```python
from build123d import *

# Parameters (mm, degrees)
SKETCH1_W           = 30
SKETCH1_H           = 42
BOSS_EXTRUDE1_DEPTH = 13.5
SKETCH2_R           = 11
CUT_EXTRUDE1_DEPTH  = 38.349698794
SKETCH3_R           = 1.9
CUT_EXTRUDE2_DEPTH  = 10
SKETCH7_W           = 27
SKETCH7_H           = 42
BOSS_EXTRUDE2_DEPTH = 4.4
SKETCH6_R           = 1.9
CUT_EXTRUDE3_DEPTH  = 10
FILLET1_R           = 10


with BuildPart() as part:
    # Sketch1 → Boss-Extrude1 (new, symmetric)
    with BuildSketch(Plane.XY):
        Rectangle(SKETCH1_W, SKETCH1_H)
    extrude(amount=BOSS_EXTRUDE1_DEPTH, both=True)

    # Sketch2 → Cut-Extrude1 (cut, through all)
    with BuildSketch(Plane.XY.offset(13.5)):
        Circle(SKETCH2_R)
    extrude(amount=-CUT_EXTRUDE1_DEPTH, mode=Mode.SUBTRACT)

    # Sketch3 → Cut-Extrude2 (cut)
    with BuildSketch(Plane.XY.offset(13.5)):
        with Locations((-11.313708499, 11.313708499)):
            Circle(SKETCH3_R)
        with Locations((0, 16)):
            Circle(SKETCH3_R)
        with Locations((11.313708499, 11.313708499)):
            Circle(SKETCH3_R)
        with Locations((11.313708499, -11.313708499)):
            Circle(SKETCH3_R)
        with Locations((0, -16)):
            Circle(SKETCH3_R)
        with Locations((-11.313708499, -11.313708499)):
            Circle(SKETCH3_R)
    extrude(amount=-CUT_EXTRUDE2_DEPTH, mode=Mode.SUBTRACT)

    # Sketch7 → Boss-Extrude2 (add)
    with BuildSketch(Plane(origin=(15, 0, 0), x_dir=(0, 0, -1), z_dir=(1, 0, 0))):
        Rectangle(SKETCH7_W, SKETCH7_H)
    extrude(amount=BOSS_EXTRUDE2_DEPTH)

    # Sketch6 → Cut-Extrude3 (cut)
    with BuildSketch(Plane(origin=(19.4, 0, 0), x_dir=(0, 0, -1), z_dir=(1, 0, 0))):
        with Locations((9.5, 17)):
            Circle(SKETCH6_R)
        with Locations((-9.5, 17)):
            Circle(SKETCH6_R)
        with Locations((9.5, -17)):
            Circle(SKETCH6_R)
        with Locations((-9.5, -17)):
            Circle(SKETCH6_R)
    extrude(amount=-CUT_EXTRUDE3_DEPTH, mode=Mode.SUBTRACT)

    # Fillet1
    fillet1_edges = [part.edges().sort_by_distance(p)[0] for p in [
        (-15, -21, 0),
        (-15, 21, 0),
    ]]
    fillet(fillet1_edges, radius=FILLET1_R)


solid = part.part
```
Verification items for the finished model (mm, model axes). A direction names the side the tool comes from. Coordinates: 2 decimals unless noted, no trailing zeros. Loops run counter-clockwise (first coordinate to the right, second up) from the corner with the lowest first, then second, coordinate; pieces in that order, holes last. Notation, with made-up numbers: (69, -6.5) - (110, -6.5) arc R19 ccw to (110, 9.5) - close; hole circle Ø3 at (58, -23). An arc over 180 degrees is marked (long way). Answer as a JSON object with one key per item and string values.
(1) Mould release check, pull along Y, two halves, no side actions. Record for faces 4 (the cylindrical face through (-0.247, 17.884, 8.57)), 5 (the flat face through (-15, 0, 0)), 6 (the cylindrical face through (-12.15, -17.99, 0.19)): pulls with the +Y half, pulls with the -Y half, needs draft (parallel to the pull), parting line crosses it, or undercut.
Response:
{"face 4": "undercut", "face 5": "needs draft", "face 6": "pulls with the -Y half"}
(2) Cross-section at A-A, the plane y = 0. Record the boundary of the cut face in (x, z).
Response:
{"outline": "(-15, -13.5) - (-11, -13.5) - (-11, 13.5) - (-15, 13.5) - close; (11, -13.5) - (19.4, -13.5) - (19.4, 13.5) - (11, 13.5) - close"}
(3) Cross-section at B-B, the plane z = -9.5. Record the boundary of the cut face in (x, y).
Response:
{"outline": "(-15, -11) arc R10 ccw to (-5, -21) - (19.4, -21) - (19.4, -18.9) - (9.4, -18.9) - (9.4, -15.1) - (19.4, -15.1) - (19.4, 15.1) - (9.4, 15.1) - (9.4, 18.9) - (19.4, 18.9) - (19.4, 21) - (-5, 21) arc R10 ccw to (-15, 11) - close; hole circle Ø22 at (0, 0)"}
(4) Cross-section at D-D, the plane x = 12. Record the boundary of the cut face in (y, z).
Response:
{"outline": "(-21, -13.5) - (21, -13.5) - (21, 13.5) - (13.09, 13.5) - (13.09, 3.5) - (9.54, 3.5) - (9.54, 13.5) - (-9.54, 13.5) - (-9.54, 3.5) - (-13.09, 3.5) - (-13.09, 13.5) - (-21, 13.5) - close; hole circle Ø3.8 at (-17, -9.5); hole circle Ø3.8 at (-17, 9.5); hole circle Ø3.8 at (17, -9.5); hole circle Ø3.8 at (17, 9.5)"}
(5) Cross-section at C-C, the plane x = 0. Record the boundary of the cut face in (y, z), then the cut area to 3 significant figures.
Response:
{"outline": "(-21, -13.5) - (-11, -13.5) - (-11, 13.5) - (-14.1, 13.5) - (-14.1, 3.5) - (-17.9, 3.5) - (-17.9, 13.5) - (-21, 13.5) - close; (11, -13.5) - (21, -13.5) - (21, 13.5) - (17.9, 13.5) - (17.9, 3.5) - (14.1, 3.5) - (14.1, 13.5) - (11, 13.5) - close", "area": "464 mm²"}
(6) Access from +Z, -Z, +X, -X, +Y, -Y to the whole of each face (thin tool, end or side, straight path). Record for faces 1 (the cylindrical face through (-9.559, 10.586, 8.57)), 2 (the cylindrical face through (14.47, -15.398, -10.521)), 3 (the flat face through (6, -10, 13.5)).
Response:
{"face 1": "+Z", "face 2": "+X", "face 3": "+Z, +X, -X, +Y, -Y"}
(7) Scan lines: line 1 along Y through (x, z) = (10, 9.75); line 2 along X through (y, z) = (12, 4); line 3 along Y through (x, z) = (12.5, 4). Record each from-to range of solid material in increasing order.
Response:
{"line 1": "y = -21 to -18.88, -15.12 to -12.69, -9.94 to -4.58, 4.58 to 9.94, 12.69 to 15.12, 18.88 to 21", "line 2": "x = -14.95 to -13.09, -9.54 to 9.54, 13.09 to 19.4", "line 3": "y = -21 to -12.8, -9.83 to 9.83, 12.8 to 21"}
(8) Go/stop test with flat-tipped pins: pin 1 Ø4.5 at (y, z) = (-17, -9.5) entering from -X; pin 2 Ø3.5 at (y, z) = (-17, 9.5) entering from -X; pin 3 Ø1.9 at (x, y) = (11, -10.5) entering from +Z. Record where each tip stops, or that it passes through.
Response:
{"pin 1": "stops at x = -14.27", "pin 2": "stops at x = -14.05", "pin 3": "stops at z = 3.5"}
